```python
from build123d import *

# Parameters (mm, degrees)
BOSS_EXTRUDE1_DEPTH = 8
FILLET1_R           = 27.432
FILLET3_START       = -62.980474595
FILLET3_DEPTH       = 78.103235199
FILLET3_2_DEPTH     = 78.103235199
SKETCH2_R           = 3
CUT_EXTRUDE1_DEPTH  = 6


with BuildPart() as part:
    # Sketch1 → Boss-Extrude1 (new body)
    with BuildSketch(Plane(origin=(0, 0, 0), x_dir=(1, 0, 0), z_dir=(0, 1, 0))):
        with BuildLine():
            Line((-20, 20), (-55, -25))
            ThreePointArc((-55, -25), (-46.213203436, -46.213203436), (-25, -55))
            Line((-25, -55), (20, -20))
            Line((20, -20), (20, -1.082))
            ThreePointArc((20, -1.082), (13.825225161, 13.825225161), (-1.082, 20))
            Line((-1.082, 20), (-20, 20))
        make_face()
    extrude(amount=BOSS_EXTRUDE1_DEPTH)

    # Fillet1
    # the kernel refuses this fillet: 27.432 mm, written as the material it takes off along each edge
    with BuildSketch(Plane(origin=(-1.082, 0, -20), x_dir=(0, 1, 0), z_dir=(-1, 0, 0)), Plane(origin=(20, 0, 68.406611119), x_dir=(0, 1, 0), z_dir=(0, 0, -1))) as fillet1_piece_1:
        with BuildLine():
            CenterArc((27.432, -19.362644447), FILLET1_R, 135.102431051, 44.897568949)
            Line((0, -19.362644447), (-0.54864, -19.362644447))
            Line((-0.54864, -19.362644447), (-0.54864, 0))
            Line((-0.54864, 0), (0, 0.54864))
            ThreePointArc((0, 0.54864), (4, 0.54864), (7.61136, 0.387252889))
            Line((7.61136, 0.387252889), (8, 0))
        make_face()
    extrude(amount=67.324611119, mode=Mode.SUBTRACT)
    with BuildSketch(Plane(origin=(-1.082, 0, 1.082), x_dir=(1, 0, 0), z_dir=(0, 0, 1))) as fillet1_piece_2:
        with BuildLine():
            CenterArc((1.719355553, 27.432), FILLET1_R, 270, 44.897568949)
            Line((1.719355553, 0), (1.719355553, -0.54864))
            Line((1.719355553, -0.54864), (21.082, -0.54864))
            Line((21.082, -0.54864), (21.63064, 0))
            ThreePointArc((21.63064, 0), (21.63064, 4), (21.469252889, 7.61136))
            Line((21.469252889, 7.61136), (21.082, 8))
        make_face()
    revolve(axis=Axis((-1.082, 0, 1.082), (0, 1, 0)), revolution_arc=90, mode=Mode.SUBTRACT)

    # Fillet3: read off the stored shape, not the designer's step
    # Fillet3 outline → Fillet3 (cut)
    with BuildSketch(Plane(origin=(0, 0, 0), x_dir=(0.7893522173763267, 0, 0.6139406135149199), z_dir=(0.6139406135149199, 0, -0.7893522173763268)).offset(FILLET3_START)):
        with BuildLine():
            ThreePointArc((-28.065856618, -8), (-22.900060751, -2.167840434), (-15.416745977, 0))
            Line((-15.416745977, 0), (-28.065856618, 0))
            Line((-28.065856618, 0), (-28.065856618, -8))
        make_face()
    extrude(amount=FILLET3_DEPTH, mode=Mode.SUBTRACT)

    # Fillet3 2 outline → Fillet3 2 (cut)
    with BuildSketch(Plane(origin=(0, 0, 0), x_dir=(0.6139406135149201, 0, 0.7893522173763264), z_dir=(0.7893522173763264, 0, -0.6139406135149204)).offset(FILLET3_START)):
        with BuildLine():
            Line((28.065856618, 0), (15.416745977, 0))
            ThreePointArc((15.416745977, 0), (22.900060751, -2.167840434), (28.065856618, -8))
            Line((28.065856618, -8), (28.065856618, 0))
        make_face()
    extrude(amount=FILLET3_2_DEPTH, mode=Mode.SUBTRACT)

    # Sketch2 → Cut-Extrude1 (cut)
    with BuildSketch(Plane(origin=(0, 8, 0), x_dir=(1, 0, 0), z_dir=(0, 1, 0))):
        with Locations(Location((-22.88, -2.01, 0), (0, 0, 270))):
            Circle(SKETCH2_R)
        with Locations(Location((-2.01, -22.88, 0), (0, 0, 270))):
            Circle(SKETCH2_R)
    extrude(amount=-CUT_EXTRUDE1_DEPTH, mode=Mode.SUBTRACT)


solid = part.part
```
Here's how the part is built. I have some questions about the finished solid (model axes, mm). A direction names the side the tool comes from. Give positions to 0.01 mm unless a question says otherwise; leave off trailing zeros. Answer as a JSON object with one key per item and string values. Group by question number.
Item 1: For P1, Ø2, axis at x = -28.5, y = 5.5, coming from the -Z side; P2, Ø4, axis at y = 4.5, z = -11.5, coming from the -X side; P3, Ø1.5, axis at x = -21.5, y = 4, coming from the -Z side, each with a flat end and sliding along its axis, tell me the tip position at first contact or that it passes through.
Item 2: Which directions (+Z, -Z, +X, -X, +Y, -Y) give clear straight access to the entire face, cutting with the end or side of a thin tool? Please do faces 5 (the flat face through (-25, 0, 25)), 6 (the cylindrical face through (-20.85, 5.04, -0.2)).
Item 3: Please list where these lines run through material, in increasing order: probe 1 along X at (y, z) = (4.55, 2.01); probe 2 along X at (y, z) = (3.7, 2.01); probe 3 along X at (y, z) = (6.25, 28.5).
Item 4: If we section it at A-A on y = 3: Give the number of separate pieces and of enclosed holes in the cut face, and give its area (3 significant figures).
Item 5: If we mould it in two halves opening along X, with no side actions, what happens to faces 1 (the flat face through (-23, 2, 2)), 2 (the cylindrical face through (-9.8, 2.1, 36.5)), 3 (the flat face through (-18, 8, 17)), 4 (the cylindrical face through (-46.445, 3.944, 45.979))? For each: pulls with the +X half, pulls with the -X half, needs draft (parallel to the pull), parting line crosses it, or undercut.
Result set:
{
 "1": {"P1": "z = -8.33", "P2": "x = -26.17", "P3": "z = -14.95"},
 "2": {"face 5": "+Z, -Z, +X, -X, -Y", "face 6": "+Y"},
 "3": {"probe 1": "-34.18 to -25.88, -19.88 to 15.77", "probe 2": "-33.11 to -25.88, -19.88 to 14.4", "probe 3": "-54.8 to 7.46"},
 "4": {"separate pieces": "1", "enclosed holes": "2", "area": "2,800 mm²"},
 "5": {"face 1": "undercut", "face 2": "pulls with the +X half", "face 3": "needs draft", "face 4": "pulls with the -X half"}
}
